Could you check a few things on this model? Use its own coordinates, in mm. Coordinates: 2 decimals unless noted, no trailing zeros. Write each loop counter-clockwise with the first axis right and the second up, starting at its lowest first coordinate (ties: lowest second). Pieces come first, ordered by that corner, then holes.
```python
from build123d import *

# Parameters (mm, degrees)
SKETCH1_W          = 5.5
SKETCH1_H          = 0.3
SKETCH2_R          = 1
CUT_EXTRUDE1_DEPTH = 10
FILLET1_R          = 1


with BuildPart() as part:
    # Sketch1 → Revolve1 (revolve)
    with BuildSketch(Plane.XY, mode=Mode.PRIVATE) as revolve1_sk:
        with Locations((-9.75, 0.15)):
            Rectangle(SKETCH1_W, SKETCH1_H)
    revolve(revolve1_sk.sketch.rotate(Axis((0, 0, 0), (0, 1, 0)), 270), axis=Axis((0, 0, 0), (0, 1, 0)))

    # Sketch2 → Cut-Extrude1 (cut)
    with BuildSketch(Plane(origin=(0, 0.3, 0), x_dir=(1, 0, 0), z_dir=(0, 1, 0))):
        with Locations((4.571073678, -5)):
            Circle(SKETCH2_R)
        with Locations((11.589188307, 4.5)):
            Circle(SKETCH2_R)
    extrude(amount=-CUT_EXTRUDE1_DEPTH, mode=Mode.SUBTRACT)

    # Fillet1
    fillet1_edges = [part.edges().sort_by_distance(p)[0] for p in [
        (5.405006845, 0.15, 4.448134553),
        (3.946825109, 0.15, 5.781225783),
        (11.976907898, 0.15, -3.578222631),
        (11.253259969, 0.15, -5.441887547),
    ]]
    fillet(fillet1_edges, radius=FILLET1_R)


solid = part.part
```
1. Please list where these lines run through material, in increasing order: line 1 along Z through (x, y) = (0, 0.15); line 2 along Z through (x, y) = (-6.25, 0.25).
Verdict:
line 1: z = -12.5 to -7, 7 to 12.5
line 2: z = -10.83 to -3.15, 3.15 to 10.83
2. I want a section at B-B on x = 0. Please give me the cut outline in (y, z).
Verdict:
outline: (0, -12.5) - (0.3, -12.5) - (0.3, -7) - (0, -7) - close; (0, 7) - (0.3, 7) - (0.3, 12.5) - (0, 12.5) - close
3. I want a section at C-C on x = 10. Please give me the cut outline in (y, z).
Verdict:
outline: (0, -7.5) - (0.3, -7.5) - (0.3, 7.5) - (0, 7.5) - close
4. I want a section at A-A on z = 0. Please give me the cut outline in (x, y), plus the area to 3 significant figures.
Verdict:
outline: (-12.5, 0) - (-7, 0) - (-7, 0.3) - (-12.5, 0.3) - close; (7, 0) - (12.5, 0) - (12.5, 0.3) - (7, 0.3) - close
area: 3.30 mm2
